Model file for the job. Use its own axes, mm. Face numbers are marked on the shaded views. A direction names the side the tool comes from. Give positions to 0.01 mm unless a question says otherwise; leave off trailing zeros. Order: outer loops, then holes, each group sorted by start corner. A loop starts at its lowest first (then second) coordinate and runs counter-clockwise, first axis right, second up. Notation, with made-up numbers: (68.5, 43) - (98.5, 43) arc R14 ccw to (98.5, 57) - close; hole circle Ø8 at (-27, -13.75). An arc over 180 degrees is marked (long way). Use CSV: the item, a comma, the result in double quotes. Start each with the question number.
(1) Pull direction X, two halves, no side cores. Call the marked faces 3, 4 and 5: +X half, -X half, draft (parallel to the pull), parting line (faces both ways), or undercut.
(2) Band-saw the part on A-A, the plane x = 0. Give the cut face in (y, z), then the cut area to 3 significant figures.
(3) Drop flat-ended pins along their axis: pin 1 Ø5 at (x, z) = (3, 8) entering from +Y; pin 2 Ø10 at (x, z) = (-7.5, -3) entering from +Y. Give the stop position or say it passes through.
(4) Probe L1, parallel to Z at x = -4, y = 8.5; L2, parallel to X at y = 0.3, z = 0; L3, parallel to X at y = 7.75, z = 9.5. List the from-to ranges inside material, lowest first.
(5) Band-saw the part on B-B, the plane y = 7.25. Give the cut face in (x, z), then the cut area to 3 significant figures.
(6) Tool access for the marked faces 1 and 2: list every direction of +Z, -Z, +X, -X, +Y, -Y with a clear straight run to the whole face (end or side of a thin tool).
(7) Band-saw the part on C-C, the plane z = 0. Give the cut face in (x, y).
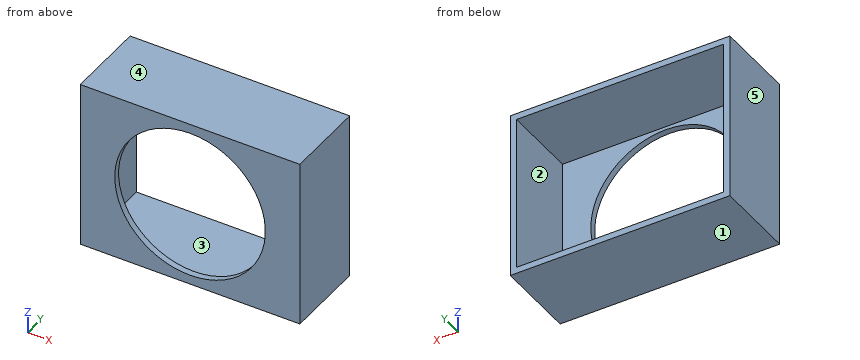
from build123d import *

# Parameters (mm, degrees)
SKETCH_1_W          = 35
SKETCH_1_H          = 27
EXTRUDE_1_DEPTH     = 13
CUT_EXTRUDE_START   = 1
SKETCH_2_W          = 33
SKETCH_2_H          = 25
CUT_EXTRUDE_1_DEPTH = 15
SKETCH_3_R          = 12
CUT_EXTRUDE_2_DEPTH = 26.64176281


with BuildPart() as part:
    # 스케치1 → 보스-돌출1 (new body)
    with BuildSketch(Plane(origin=(0, 0, 0), x_dir=(1, 0, 0), z_dir=(0, 1, 0))):
        Rectangle(SKETCH_1_W, SKETCH_1_H)
    extrude(amount=EXTRUDE_1_DEPTH)

    # 스케치2 → 컷-돌출1 (cut)
    with BuildSketch(Plane(origin=(0, 0, 0), x_dir=(1, 0, 0), z_dir=(0, 1, 0)).offset(CUT_EXTRUDE_START)):
        Rectangle(SKETCH_2_W, SKETCH_2_H)
    extrude(amount=CUT_EXTRUDE_1_DEPTH, mode=Mode.SUBTRACT)

    # 스케치3 → 컷-돌출2 (cut, through all)
    with BuildSketch(Plane(origin=(0, 0, 0), x_dir=(1, 0, 0), z_dir=(0, 1, 0))):
        with Locations(Location((0, 0, 0), (0, 0, 90))):
            Circle(SKETCH_3_R)
    extrude(amount=CUT_EXTRUDE_2_DEPTH, mode=Mode.SUBTRACT)


solid = part.part
Answer block:
1,face 3,"undercut"
1,face 4,"draft"
1,face 5,"-X half"
2,outline,"(0, -13.5) - (13, -13.5) - (13, -12.5) - (1, -12.5) - (1, -12) - (0, -12) - close; (0, 12) - (1, 12) - (1, 12.5) - (13, 12.5) - (13, 13.5) - (0, 13.5) - close"
2,area,"27.0 mm2"
3,pin 1,"passes through"
3,pin 2,"stops at y = 1"
4,L1,"z = -13.5 to -12.5, 12.5 to 13.5"
4,L2,"x = -17.5 to -12, 12 to 17.5"
4,L3,"x = -17.5 to -16.5, 16.5 to 17.5"
5,outline,"(-17.5, -13.5) - (17.5, -13.5) - (17.5, 13.5) - (-17.5, 13.5) - close; hole (-16.5, -12.5) - (16.5, -12.5) - (16.5, 12.5) - (-16.5, 12.5) - close"
5,area,"120 mm2"
6,face 1,"-Z, +X, -X, +Y, -Y"
6,face 2,"+Y"
7,outline,"(-17.5, 0) - (-12, 0) - (-12, 1) - (-16.5, 1) - (-16.5, 13) - (-17.5, 13) - close; (12, 0) - (17.5, 0) - (17.5, 13) - (16.5, 13) - (16.5, 1) - (12, 1) - close"
